For this review, use the dimensioned drawing (mm, ordinates from the lowest corner) and the shaded views. A direction names the side the tool comes from. Round coordinates to 2 decimals unless told otherwise and drop trailing zeros. Loops run counter-clockwise (first coordinate to the right, second up) from the corner with the lowest first, then second, coordinate; pieces in that order, holes last. Notation, with made-up numbers: M 31.25,86.5 L 88.25,86.5 A22 cw 88.25,103.5 Z; hole C 68,62.5 d7. An arc over 180 degrees is marked long. Use a Markdown table: item, result. Add a question column.
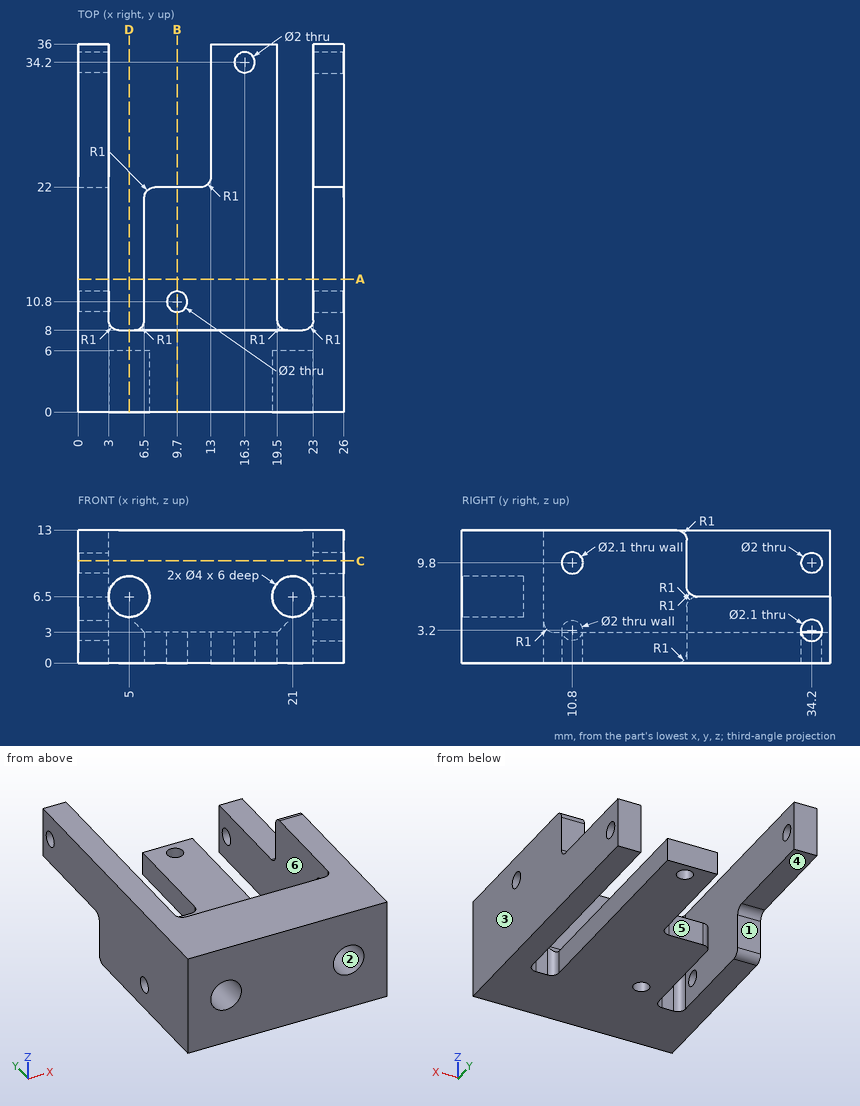
(1) Consider section C-C, the plane z = 10. Give the boundary of the cut face in (x, y).
(2) Insertion check: pin 1 Ø2.5 at (x, y) = (25, 29.5) entering from +Z; pin 2 Ø6.5 at (x, y) = (14.5, 19.5) entering from +Z; pin 3 Ø2 at (x, z) = (20.5, 11.5) entering from +Y; pin 4 Ø5 at (y, z) = (30.5, 5) entering from -X. Each pin has a flat end and moves straight along its axis. Give the tip position at first contact, or say it passes through.
(3) To check wall thickness, follow probe 1 along X at (y, z) = (3.1, 6.5); probe 2 along Z at (x, y) = (5, 4.5); probe 3 along X at (y, z) = (15, 12.25). State the ranges of each line that lie inside material, in increasing order.
(4) For the marked faces 4, 5 and 6, list the 3-axis set-ups (+Z, -Z, +X, -X, +Y, -Y) from which the entire face can be reached by the end or side of a thin tool; tool diameter is ignored.
(5) Consider section A-A, the plane y = 13. Give the boundary of the cut face in (x, z), then the cut area to 3 significant figures.
(6) Consider section B-B, the plane x = 9.7. Give the boundary of the cut face in (y, z), then the cut area to 3 significant figures.
(7) Consider section D-D, the plane x = 5. Give the boundary of the cut face in (y, z).
(8) Draft analysis for pull direction X (two halves, no side actions). For the marked faces 1, 2 and 3, state which applies: released by +X, released by -X, zero draft, split by the parting line, or undercut.
Found:
| question | item | result |
|---|---|---|
| 1 | outline | M 0,0 L 26,0 L 26,9.77 L 23,9.77 L 23,9 A1 cw 22,8 L 4,8 A1 cw 3,9 L 3,33.22 L 0,33.22 Z; M 0,35.18 L 3,35.18 L 3,36 L 0,36 Z; M 23,11.83 L 26,11.83 L 26,22 L 23,22 Z |
| 2 | pin 1 | stops at z = 6.5 |
| 2 | pin 2 | stops at z = 3 |
| 2 | pin 3 | stops at y = 8 |
| 2 | pin 4 | stops at x = 0 |
| 3 | probe 1 | x = 0 to 3, 7 to 19, 23 to 26 |
| 3 | probe 2 | z = 0 to 4.5, 8.5 to 13 |
| 3 | probe 3 | x = 0 to 3, 23 to 26 |
| 4 | face 4 | -Z, -X, +Y |
| 4 | face 5 | +Z, -Z, -X, +Y |
| 4 | face 6 | +Z, -Z, +Y |
| 5 | outline | M 0,0 L 3,0 L 3,13 L 0,13 Z; M 6.5,0 L 19.5,0 L 19.5,3 L 6.5,3 Z; M 23,0 L 26,0 L 26,13 L 23,13 Z |
| 5 | area | 117 mm^2 |
| 6 | outline | M 0,0 L 9.8,0 L 9.8,3 L 9,3 A1 cw 8,4 L 8,13 L 0,13 Z; M 11.8,0 L 22,0 L 22,3 L 11.8,3 Z |
| 6 | area | 140 mm^2 |
| 7 | outline | M 0,0 L 8,0 L 8,13 L 0,13 L 0,8.5 L 6,8.5 L 6,4.5 L 0,4.5 Z |
| 8 | face 1 | zero draft |
| 8 | face 2 | undercut |
| 8 | face 3 | released by +X |
